For this review, use the dimensioned drawing (mm, ordinates from the lowest corner) and the shaded views. Round coordinates to 2 decimals unless told otherwise and drop trailing zeros. Write each loop counter-clockwise with the first axis right and the second up, starting at its lowest first coordinate (ties: lowest second). Pieces come first, ordered by that corner, then holes. Notation, with made-up numbers: M 73.25,46.5 L 123.25,46.5 A21 cw 123.25,65.5 Z; hole C -33.75,-29 d8. An arc over 180 degrees is marked long. Answer in a Markdown table with one row per item.
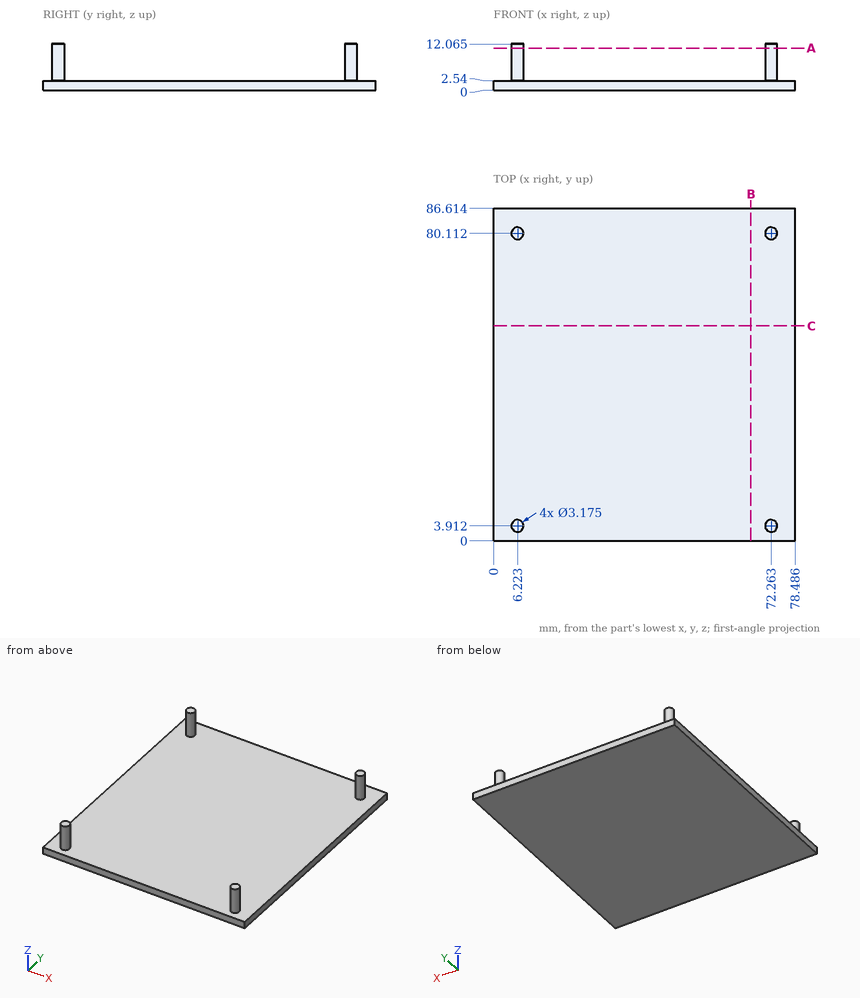
Q1. For probe 1 along Z at (x, y) = (45.5, 15.5), list the stretches that pass through material, from the lowest coordinate up.
Found:
| item | result |
|---|---|
| probe 1 | 0 to 2.54 |
Q2. Take a section at C-C (y = 56). State the section outline as (x, z) points, then the cut area to 3 significant figures.
Found:
| item | result |
|---|---|
| outline | M 0,0 L 78.49,0 L 78.49,2.54 L 0,2.54 Z |
| area | 199 mm² |
Q3. Take a section at A-A (z = 11). State how many separate pieces and enclosed holes the cut face has.
Found:
| item | result |
|---|---|
| separate pieces | 4 |
| enclosed holes | 0 |
Q4. Insertion check: P1, Ø3, axis at x = 42.5, y = 75, coming from the +Z side; P2, Ø6, axis at y = 44.5, z = 6, coming from the -X side. Each pin has a flat end and moves straight along its axis. Give the tip position at first contact, or say it passes through.
Found:
| item | result |
|---|---|
| P1 | z = 2.54 |
| P2 | through |
Q5. Take a section at B-B (x = 67). State the section outline as (y, z) points, then the cut area to 3 significant figures.
Found:
| item | result |
|---|---|
| outline | M 0,0 L 86.61,0 L 86.61,2.54 L 0,2.54 Z |
| area | 220 mm² |
